Model file for the job. Use its own axes, mm. Face numbers are marked on the shaded views. A direction names the side the tool comes from. Round coordinates to 2 decimals unless told otherwise and drop trailing zeros. Loops run counter-clockwise (first coordinate to the right, second up) from the corner with the lowest first, then second, coordinate; pieces in that order, holes last. Notation, with made-up numbers: (5, -16.75) - (58, -16.75) arc R38 ccw to (58, 22.25) - close; hole circle Ø6 at (85, -4). An arc over 180 degrees is marked (long way). Use one line per item in the form item = value.
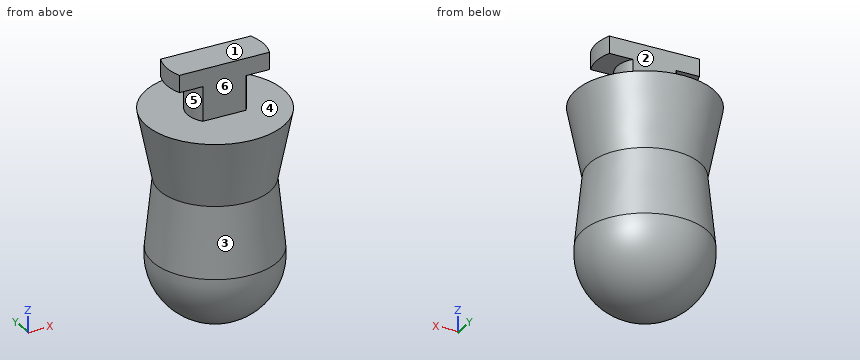
from build123d import *

# Parameters (mm, degrees)
F3_DEPTH = 9.525


with BuildPart() as f1:
    # F0 (on Front) → F1 (revolve)
    with BuildSketch(Plane.XZ):
        Polygon((0, -12.7), (0, 0), (-5.08, 0), (-12.7, 0), (-10.16, -12.7), align=None)
        Polygon((-5.08, 0), (0, 0), (0, 9.525), (-8.89, 9.525), (-8.89, 6.35), (-5.08, 6.35), align=None)
        Polygon((0, -25.4), (0, -12.7), (-10.16, -12.7), (-11.4633519053, -25.4), align=None)
        with BuildLine():
            Line((0, -38.1), (0, -25.4))
            Line((0, -25.4), (-11.4633519053, -25.4))
            ThreePointArc((-11.4633519053, -25.4), (-8.5542158744, -34.2976982984), (0, -38.1))
        make_face()
    revolve(axis=Axis((0, 0, -19.05), (0, 0, -1)))

    # F2 (on face) → F3 (cut, through all)
    with BuildSketch(Plane.XY.offset(9.525)):
        with BuildLine():
            ThreePointArc((8.3037024874, 3.175), (0, 8.89), (-8.3037024874, 3.175))
            Line((-8.3037024874, 3.175), (8.3037024874, 3.175))
        make_face()
        with BuildLine():
            Line((8.3037024874, -3.175), (-8.3037024874, -3.175))
            ThreePointArc((-8.3037024874, -3.175), (0, -8.89), (8.3037024874, -3.175))
        make_face()
        with BuildLine():
            ThreePointArc((10.9695693512, 3.175), (0, 11.4198107144), (-10.9695693512, 3.175))
            Line((-10.9695693512, 3.175), (-8.3037024874, 3.175))
            ThreePointArc((-8.3037024874, 3.175), (0, 8.89), (8.3037024874, 3.175))
            Line((8.3037024874, 3.175), (10.9695693512, 3.175))
        make_face()
        with BuildLine():
            Line((-8.3037024874, -3.175), (-10.9695693512, -3.175))
            ThreePointArc((-10.9695693512, -3.175), (0, -11.4198107144), (10.9695693512, -3.175))
            Line((10.9695693512, -3.175), (8.3037024874, -3.175))
            ThreePointArc((8.3037024874, -3.175), (0, -8.89), (-8.3037024874, -3.175))
        make_face()
        with BuildLine():
            Line((-8.3037024874, 3.175), (-10.9695693512, 3.175))
            ThreePointArc((-10.9695693512, 3.175), (-11.4198107144, 0), (-10.9695693512, -3.175))
            Line((-10.9695693512, -3.175), (-8.3037024874, -3.175))
            ThreePointArc((-8.3037024874, -3.175), (-8.89, 0), (-8.3037024874, 3.175))
        make_face()
        with BuildLine():
            ThreePointArc((11.4198107144, 0), (11.3066901072, 1.6033825405), (10.9695693512, 3.175))
            Line((10.9695693512, 3.175), (8.3037024874, 3.175))
            ThreePointArc((8.3037024874, 3.175), (8.7421969525, 1.6143396307), (8.89, 0))
            ThreePointArc((8.89, 0), (8.7421969525, -1.6143396307), (8.3037024874, -3.175))
            Line((8.3037024874, -3.175), (10.9695693512, -3.175))
            ThreePointArc((10.9695693512, -3.175), (11.3066901072, -1.6033825405), (11.4198107144, 0))
        make_face()
    extrude(amount=-F3_DEPTH, mode=Mode.SUBTRACT)


solid = f1.part
1. Cut at D-D, the plane z = -27.5. Give the cut face in (x, y).
Geometry check:
outline = circle Ø22.97 at (0, 0)
2. Wall check: probe 1 along Y at (x, z) = (2.75, 7) (3 decimals); probe 2 along Y at (x, z) = (4, -0.5); probe 3 along Z at (x, y) = (-7, -5.75). Give the ranges that are in metal, low to high.
Geometry check:
probe_1 = -3.175 to 3.175
probe_2 = -11.95 to 11.95
probe_3 = -33.7 to 0
3. Pull direction Z, two halves, no side cores. Call the marked faces 1, 2 and 3: +Z half, -Z half, draft (parallel to the pull), parting line (faces both ways), or undercut.
Geometry check:
face_1 = +Z half
face_2 = draft
face_3 = undercut
4. Cut at C-C, the plane z = -35. Give the cut face in (x, y).
Geometry check:
outline = circle Ø15.73 at (0, 0)
5. Flat gauge pins, fed straight in: pin 1 (6 mm diameter, centred on x = -9.5, y = -9, fed in from +Z); pin 2 (4 mm diameter, centred on x = 6, y = -0.5, fed in from -Z); pin 3 (5 mm diameter, centred on x = -3, z = 3.5, fed in from -Y) (3 decimals); pin 4 (1 mm diameter, centred on x = 9.5, y = -10, fed in from -Z). Where does each tip first touch, or does it go through?
Geometry check:
pin_1 = 0
pin_2 = -37.38
pin_3 = -3.175
pin_4 = through
6. Cut at B-B, the plane x = 0. Give the cut face in (y, z) (3 decimals).
Geometry check:
outline = (-12.7, 0) - (-10.16, -12.7) - (-11.463, -25.4) arc R11.524 ccw (long way) to (11.463, -25.4) - (10.16, -12.7) - (12.7, 0) - (3.175, 0) - (3.175, 9.525) - (-3.175, 9.525) - (-3.175, 0) - close
7. Tool access for the marked faces 4, 5 and 6: list every direction of +Z, -Z, +X, -X, +Y, -Y with a clear straight run to the whole face (end or side of a thin tool).
Geometry check:
face_4 = none
face_5 = -X
face_6 = +Z, +X, -X, -Y
8. Cut at A-A, the plane y = 0. Give the cut face in (x, z) (3 decimals).
Geometry check:
outline = (-12.7, 0) - (-10.16, -12.7) - (-11.463, -25.4) arc R11.524 ccw (long way) to (11.463, -25.4) - (10.16, -12.7) - (12.7, 0) - (5.08, 0) - (5.08, 6.35) - (8.89, 6.35) - (8.89, 9.525) - (-8.89, 9.525) - (-8.89, 6.35) - (-5.08, 6.35) - (-5.08, 0) - close
